Can you work these out from the model? Positions are in its coordinate system, mm. A direction names the side the tool comes from. Give positions to 0.01 mm unless a question says otherwise; leave off trailing zeros. Order: outer loops, then holes, each group sorted by start corner. A loop starts at its lowest first (then second) coordinate and runs counter-clockwise, first axis right, second up. Notation, with made-up numbers: M -5,81.5 L 12,81.5 A28 ccw 12,113.5 Z; hole C 67,-0.75 d7. An arc over 180 degrees is marked long. Use one line per item in the form item = value. Start each with the question number.
1. I need wall thicknesses on L1, parallel to Y at x = 0, z = -4; L2, parallel to Z at x = 9, y = 1; L3, parallel to Y at x = 0, z = -10.75. Which ranges of each line are inside material? Lowest first, please.
2. I want a section at A-A, the plane y = 0. List the corners of the cut face in (x, z) for me (3 decimals).
3. We'd pull the mould along Y, two halves only. Please class faces 1 (the face through (0, 5, 0)), 2 (the face through (0.53, -11.99, -5.32)), 3 (the face through (0.867, -3.905, -8.112)): +Y half, -Y half, draft (parallel to the pull), parting line (faces both ways), or undercut.
4. Will these pins go through, and if not, where does the flat tip stop? P1, Ø5, axis at x = 4.5, z = -12, coming from the +Y side; P2, Ø1.5, axis at x = -11, z = -15.5, coming from the -Y side; P3, Ø9.5, axis at x = -3.5, y = 3.5, coming from the -Z side.
5. For faces 4 (the face through (4, 2, -16)), 5 (the face through (-11.9, -2.7, -10.2)), which set-ups out of +Z, -Z, +X, -X, +Y, -Y let a thin tool reach every point of the face, with its end or its side?
6. I want a section at D-D, the plane z = -12.25. List the corners of the cut face in (x, y) for me, and give its area (3 significant figures).
7. I want a section at C-C, the plane z = -7.5. List the corners of the cut face in (x, y) for me, and give its area (3 significant figures).
Autodesk Inventor part; units mm, degrees
ref_plane "YZ Plane" through (0, 0, 0) normal (1, 0, 0) x (0, 1, 0)
ref_plane "XZ Plane" through (0, 0, 0) normal (0, 1, 0) x (-1, 0, 0)
ref_plane "XY Plane" through (0, 0, 0) normal (0, 0, 1) x (1, 0, 0)
sketch "Sketch1" plane through (0, 0, 0) normal (1, 0, 0) x (0, 1, 0)
  line L0 (0, 0) -> (12, 0)
  line L1 (12, 0) -> (12, -10)
  line L2 (12, -10) -> (15.63, -13.63)
  line L3 (15.63, -13.63) -> (11.1401, -17.61)
  line L4 (11.1401, -17.61) -> (9.515, -16)
  line L5 (9.515, -16) -> (0, -16)
  line L6 (0, -16) -> (0, 0)
  dimension "d0" = 12
  dimension "d1" = 10
  dimension "d2" = 15.63
  dimension "d3" = 13.63
  dimension "d4" = 17.61
  dimension "d5" = 6
  dimension "d6" = 9.515
  dimension "d7" = 16
revolve "Revolution1" add sketch "Sketch1" angle 360 about axis through (0, 0, -16) along (0, 0, 1)
chamfer "Chamfer1" distance 0.5 angle 45 1 edges at (0, -12, 0)
sketch "Sketch2" plane through (0, 0, -16) normal (0, 0, -1) x (-1, 0, 0)
  circle A0 centre (0, 0) radius 4
  dimension "d12" = 8
extrude "Extrusion1" cut sketch "Sketch2" against normal up to next
equation "\"d0\" = 0.5 * Be"
equation "\"d1\" = He"
equation "\"d2\" = 0.5 * De"
equation "\"d3\" = Ge"
equation "\"d4\" = Fe"
equation "\"d5\" = Je"
equation "\"d6\" = 0.5 * Ke"
equation "\"d7\" = Le"
equation "\"d12\" = Ae"
equation "\"Ae\" = 8"
equation "\"Be\" = 24"
equation "\"De\" = 31.26"
equation "\"Ee\" = 28"
equation "\"Fe\" = 17.61"
equation "\"Ge\" = 13.63"
equation "\"He\" = 10"
equation "\"Je\" = 6"
equation "\"Ke\" = 19.03"
equation "\"Le\" = 16"
properties part number "Engrenage_spiro_conique"
Check result:
q1.L1 = -12 to -4, 4 to 12
q1.L2 = -16 to 0
q1.L3 = -12.75 to -4, 4 to 12.75
q2.outline = M -15.63,-13.63 L -11.14,-17.61 L -9.515,-16 L -4,-16 L -4,0 L -11.5,0 L -12,-0.5 L -12,-10 Z; M 4,-16 L 9.515,-16 L 11.14,-17.61 L 15.63,-13.63 L 12,-10 L 12,-0.5 L 11.5,0 L 4,0 Z
q3.face_1 = draft
q3.face_2 = parting line
q3.face_3 = undercut
q4.P1 = 15.41
q4.P2 = -9.5
q4.P3 = -16.18
q5.face_4 = -Z
q5.face_5 = +Z
q6.outline = C 0,0 d28.5; hole C 0,0 d8
q6.area = 588 mm2
q7.outline = C 0,0 d24; hole C 0,0 d8
q7.area = 402 mm2
